Autodesk Inventor part; units mm, degrees
ref_plane "YZ Plane" through (0, 0, 0) normal (1, 0, 0) x (0, 1, 0)
ref_plane "XZ Plane" through (0, 0, 0) normal (0, 1, 0) x (-1, 0, 0)
ref_plane "XY Plane" through (0, 0, 0) normal (0, 0, 1) x (1, 0, 0)
sketch "Sketch1" plane through (0, 0, 0) normal (1, 0, 0) x (0, 1, 0)
  line L0 (-45, 21) -> (45, 21)
  line L1 (45, 21) -> (45, -21)
  line L2 (-27, 21) -> (-9, 21)
  line L3 (-9, 21) -> (-9, 25)
  line L4 (-9, 25) -> (-27, 25)
  line L5 (-27, 25) -> (-27, 21)
  line L6 (9, 21) -> (27, 21)
  line L7 (27, 21) -> (27, 25)
  line L8 (27, 25) -> (9, 25)
  line L9 (9, 25) -> (9, 21)
  line L10 (-45, 10) -> (-49, 10)
  line L11 (-49, 10) -> (-49, -10)
  line L12 (-49, -10) -> (-45, -10) construction
  line L13 (-45, -10) -> (-45, 10)
  line L14 (45, 10) -> (49, 10)
  line L15 (49, 10) -> (49, -10)
  line L16 (49, -10) -> (45, -10) construction
  line L17 (45, -10) -> (45, 10)
  line L18 (-45, -21) -> (-45, 21)
  line L19 (45, 21) -> (45, -36)
  line L20 (45, -36) -> (-45, -36)
  line L21 (-45, -36) -> (-45, 21)
  line L22 (45, 10) -> (49, 10)
  line L23 (49, 10) -> (49, -20)
  line L24 (49, -20) -> (45, -20)
  line L25 (45, -20) -> (45, 10)
  line L26 (-45, 10) -> (-49, 10)
  line L27 (-49, 10) -> (-49, -20)
  line L28 (-49, -20) -> (-45, -20) construction
  line L29 (-45, -20) -> (-45, 10)
  line L30 (-18, -36) -> (-22, -36)
  line L31 (-45, -29) -> (-39, -29)
  line L32 (-39, -29) -> (-39, -25)
  line L33 (-39, -25) -> (-45, -25)
  line L34 (-45, -25) -> (-45, -29)
  line L35 (-39, -25) -> (-35, -25)
  line L36 (-35, -25) -> (-35, -33)
  line L37 (-35, -33) -> (-39, -33)
  line L38 (-39, -33) -> (-39, -25)
  line L39 (-35, -33) -> (-29, -33)
  line L40 (-29, -33) -> (-29, -29)
  line L41 (-29, -29) -> (-35, -29)
  line L42 (-35, -29) -> (-35, -33)
  line L43 (-29, -29) -> (-29, -29.15)
  line L44 (-29, -29.15) -> (-35, -29)
  line L45 (49, -20) -> (45, -20) construction
  line L46 (45, -20) -> (45, -25)
  line L47 (45, -25) -> (49, -25)
  line L48 (49, -25) -> (49, -20)
  line L49 (-45, -20) -> (-49, -20) construction
  line L50 (-49, -20) -> (-49, -25)
  line L51 (-49, -25) -> (-45, -25)
  line L52 (-45, -25) -> (-45, -20)
  line L53 (-45, -25) -> (-49, -25)
  line L54 (-49, -25) -> (-49, -20)
  line L55 (-49, -20) -> (-45, -20)
  line L56 (-45, -20) -> (-45, -25)
  point P0 (0, 0)
  point P1 (0, 21)
  point P2 (45, 0)
  point P3 (-9, 23)
  point P4 (9, 23)
  point P5 (49, 0)
  point P6 (45, -10)
  point P7 (27, 21)
  point P8 (-45, 10)
  point P9 (-45, -20)
  point P10 (-45, -20)
  point P11 (-35, -29)
  point P12 (-32, -33)
  point P13 (-32, -29)
  point P14 (-47, 10)
  point P15 (47, 10)
  dimension "d9" = 18
  dimension "d10" = 18
  dimension "d11" = 18
  dimension "d12" = 18
  dimension "d13" = 4
  dimension "d17" = 20
  dimension "d19" = 20
  dimension "d20" = 4
  dimension "d21" = 4
  dimension "d40" = 42
  dimension "d41" = 57
  dimension "d42" = 30
  dimension "d43" = 30
  dimension "d47" = 6
  dimension "d48" = 4
  dimension "d49" = 7
  dimension "d50" = 4
  dimension "d51" = 8
  dimension "d52" = 6
  dimension "d55" = 4
  dimension "d56" = 0.15
extrude "Extrusion1" add sketch "Sketch1" along normal mid plane 4 contours L0 L1 L19 L20 L21 L31 L38 L37 L39 L40 L41 L36 L35 L33 L18 L13 | L5 L4 L3 L0 | L13 L18 L55 L27 L11 L10 | L9 L8 L7 L0 | L14 L15 L23 L24 L1 | L24 L48 L47 L19 L1 | L41 L40 L44
sketch "Sketch2" plane through (2, 0, 0) normal (1, 0, 0) x (0, 0, -1)
  circle A0 centre (-11, 27) radius 2.5
  line L0 (14, -45) -> (14, -25)
  line L1 (-10, 45) -> (-21, 45)
  line L2 (6.5, -45) -> (14, -45)
  circle A1 centre (-12.5, -36.5) radius 1.55 construction
  line L3 (-21, -45) -> (-10, -45)
  line L4 (-21, 9) -> (-21, 27)
  line L5 (0, 0) -> (-4.5, 0)
  circle A2 centre (-12.5, 36.5) radius 1.55 construction
  line L6 (-14, 38) -> (-11, 38)
  line L7 (-11, 38) -> (-11, 35)
  line L8 (-11, 35) -> (-14, 35)
  line L9 (-14, 35) -> (-14, 38)
  line L10 (-14, -35) -> (-11, -35)
  line L11 (-11, -35) -> (-11, -38)
  line L12 (-11, -38) -> (-14, -38)
  line L13 (-14, -38) -> (-14, -35)
  line L14 (-25, -9) -> (-25, -27)
  line L15 (-10, -49) -> (20, -49)
  line L16 (20, -38) -> (23, -38)
  line L17 (23, -38) -> (23, -35)
  line L18 (23, -35) -> (20, -35)
  line L19 (20, -35) -> (20, -38)
  line L20 (25, -45) -> (25, -35)
  line L21 (20, 38) -> (23, 38)
  line L22 (23, 38) -> (23, 35)
  line L23 (23, 35) -> (20, 35)
  line L24 (20, 35) -> (20, 38)
  point P0 (21, 45)
  point P1 (10, 45)
  point P2 (-15.5, 45)
  point P3 (10.25, -45)
  point P4 (-15.5, -45)
  point P5 (-21, -27)
  point P6 (-12.5, 38)
  point P7 (-14, 36.5)
  point P8 (-12.5, -35)
  point P9 (-11, -36.5)
  point P10 (16.5, -49)
  point P11 (25, -49)
  point P12 (20, -36.5)
  point P13 (20, 36.5)
  dimension "d24" = 5
  dimension "d25" = 25
  dimension "d26" = 18
  dimension "d33" = 3.1
  dimension "d36" = 3
  dimension "d37" = 3
  dimension "d38" = 3
  dimension "d53" = 11
  dimension "d54" = 11
  dimension "d57" = 3
  dimension "d58" = 3
  dimension "d59" = 2
extrude "Extrusion2" cut sketch "Sketch2" against normal up to surface (4 mm away)
equation "\"d9\" = 0.2 * d3"
equation "\"d10\" = d9"
equation "\"d11\" = d9"
equation "\"d17\" = d19"
equation "\"d20\" = d13"
equation "\"d21\" = d13"
equation "\"d54\" = d53"
properties part number "Side"
Design review of the part built by this model. Coordinates are the model's own, in mm. A direction names the side the tool comes from. Coordinates: 2 decimals unless noted, no trailing zeros. Order: outer loops, then holes, each group sorted by start corner. A loop starts at its lowest first (then second) coordinate and runs counter-clockwise, first axis right, second up.
1) Wall thickness on line 1 along Z through (x, y) = (-0.55, 40); line 2 along Y through (x, z) = (1.65, 15); line 3 along Z through (x, y) = (1.4, 28): over which ranges is each line inside the solid? List them lowest first.
2) Take a section at A-A, the plane y = -31. Give the boundary of the cut face in (x, z).
3) Clearance check with flat-ended pins moving along their axes: pin 1 (2 mm diameter, centred on x = 0.5, z = 15.5, fed in from -Y); pin 2 (1.5 mm diameter, centred on x = 0, y = 36, fed in from +Z); pin 3 (1.5 mm diameter, centred on x = 1, z = 16.5, fed in from +Y). State where each tip first meets the part, or that it passes through.
4) Mouldability with a two-part tool opening along Y and no side actions: class faces 1 (the flat face through (0, -47, 10)), 2 (the flat face through (0, 45, 16)), 3 (the flat face through (0, 9, 23)), 4 (the flat face through (0, 38, 13)) as +Y half, -Y half, draft (parallel to the pull), parting line (faces both ways), or undercut.
5) Take a section at B-B, the plane z = -31. Give the boundary of the cut face in (x, y), and give its area (3 significant figures).
6) For faces 5 (the flat face through (0, -45, -23)), 6 (the flat face through (0, 47, -25)), 7 (the flat face through (0, 47, 10)), 8 (the flat face through (0, -38, -21)), 9 (the flat face through (0, -42, -29)), list the 3-axis set-ups (+Z, -Z, +X, -X, +Y, -Y) from which the entire face can be reached by the end or side of a thin tool; tool diameter is ignored.
7) Take a section at D-D, the plane x = 1.2. State how many separate pieces and enclosed holes the cut face has, and give its area (3 significant figures).
8) Take a section at C-C, the plane y = 6. Give the boundary of the cut face in (x, z).
Returned:
1. line 1: z = -36 to 21
1. line 2: y = -45 to 45
1. line 3: z = -36 to 8.71, 13.29 to 21
2. outline: (-2, -36) - (2, -36) - (2, -33) - (-2, -33) - close; (-2, -29.1) - (2, -29.1) - (2, 21) - (-2, 21) - close
3. pin 1: stops at y = -45
3. pin 2: stops at z = 21
3. pin 3: stops at y = 45
4. face 1: draft
4. face 2: +Y half
4. face 3: undercut
4. face 4: undercut
5. outline: (-2, -45) - (2, -45) - (2, -39) - (-2, -39) - close; (-2, -29) - (2, -29) - (2, 45) - (-2, 45) - close
5. area: 320 mm2
6. face 5: -Z, +X, -X, -Y
6. face 6: -Z, +X, -X, +Y
6. face 7: +Z, +X, -X, +Y
6. face 8: +X, -X
6. face 9: +X, -X, -Y
7. separate pieces: 1
7. enclosed holes: 5
7. area: 5,400 mm2
8. outline: (-2, -36) - (2, -36) - (2, 21) - (-2, 21) - close
